The model under review builds one solid part; all positions refer to its coordinate system, in mm. A direction names the side the tool comes from. Coordinates: 2 decimals unless noted, no trailing zeros. Order: outer loops, then holes, each group sorted by start corner. A loop starts at its lowest first (then second) coordinate and runs counter-clockwise, first axis right, second up. Notation, with made-up numbers: M 49,-3.5 L 100,-3.5 A19 ccw 100,14.5 Z; hole C -36.5,73.5 d8. An arc over 180 degrees is marked long. Answer in a Markdown table with one row per item.
from build123d import *

# Parameters (mm, degrees)
ESBO_O1_W                = 175
ESBO_O1_H                = 95
RESSALTO_EXTRUS_O1_DEPTH = 10
ESBO_O2_W                = 6
ESBO_O2_H                = 30
RESSALTO_EXTRUS_O2_DEPTH = 10
ESBO_O3_W                = 6
ESBO_O3_H                = 30
RESSALTO_EXTRUS_O3_DEPTH = 10
ESBO_O4_W                = 30
ESBO_O4_H                = 6
RESSALTO_EXTRUS_O4_DEPTH = 10
ESBO_O5_W                = 30
ESBO_O5_H                = 6
RESSALTO_EXTRUS_O5_DEPTH = 10
ESBO_O7_R                = 1.5
ESBO_O7_R_2              = 1.6
ESBO_O7_R_3              = 6
ESBO_O7_W                = 28.5
ESBO_O7_H                = 22.5
ESBO_O7_W_2              = 15
ESBO_O7_H_2              = 15
ESBO_O7_W_3              = 12
ESBO_O7_H_3              = 12
CORTE_EXTRUS_O2_DEPTH    = 10


with BuildPart() as part:
    # Esboço1 → Ressalto-extrusão1 (new body)
    with BuildSketch(Plane.XY):
        Rectangle(ESBO_O1_W, ESBO_O1_H)
    extrude(amount=RESSALTO_EXTRUS_O1_DEPTH)

    # Esboço2 → Ressalto-extrusão2 (add)
    with BuildSketch(Plane.ZY.offset(87.5)):
        with Locations((5, 0)):
            Rectangle(ESBO_O2_W, ESBO_O2_H)
    extrude(amount=RESSALTO_EXTRUS_O2_DEPTH)

    # Esboço3 → Ressalto-extrusão3 (add)
    with BuildSketch(Plane(origin=(87.5, 0, 0), x_dir=(0, 0, -1), z_dir=(1, 0, 0))):
        with Locations((-5, 0)):
            Rectangle(ESBO_O3_W, ESBO_O3_H)
    extrude(amount=RESSALTO_EXTRUS_O3_DEPTH)

    # Esboço4 → Ressalto-extrusão4 (add)
    with BuildSketch(Plane.XZ.offset(47.5)):
        with Locations((37.5, 5)):
            Rectangle(ESBO_O4_W, ESBO_O4_H)
        with Locations((-37.5, 5)):
            Rectangle(ESBO_O4_W, ESBO_O4_H)
    extrude(amount=RESSALTO_EXTRUS_O4_DEPTH)

    # Esboço5 → Ressalto-extrusão5 (add)
    with BuildSketch(Plane(origin=(0, 47.5, 0), x_dir=(1, 0, 0), z_dir=(0, 1, 0))):
        with Locations((0, -5)):
            Rectangle(ESBO_O5_W, ESBO_O5_H)
    extrude(amount=RESSALTO_EXTRUS_O5_DEPTH)

    # Esboço7 → Corte-extrusão2 (cut)
    with BuildSketch(Plane.XY.offset(10)):
        with Locations((73.5, -34.5)):
            Circle(ESBO_O7_R)
        with Locations((-15.5, -30.5)):
            Circle(ESBO_O7_R)
        with Locations((78.25, 7.25)):
            Circle(ESBO_O7_R_2)
        with Locations((38.25, 7.25)):
            Circle(ESBO_O7_R_2)
        with Locations((-32.5, -17.5)):
            Circle(ESBO_O7_R_3)
        Polygon((72.5, -2.5), (44, -2.5), (44, 11), (49, 17), (67.5, 17), (72.5, 11), align=None)
        with Locations((4.75, 7.25)):
            Rectangle(ESBO_O7_W, ESBO_O7_H)
        with Locations((-71.5, -38)):
            Rectangle(ESBO_O7_W_2, ESBO_O7_H_2)
        with Locations((-41.5, -38)):
            Rectangle(ESBO_O7_W_3, ESBO_O7_H_3)
    extrude(amount=-CORTE_EXTRUS_O2_DEPTH, mode=Mode.SUBTRACT)


solid = part.part
(1) Take a section at D-D (z = 3.75). State how many separate pieces and enclosed holes the cut face has, then the cut area to 3 significant figures.
Report:
| item | result |
|---|---|
| separate pieces | 1 |
| enclosed holes | 9 |
| area | 16,400 mm^2 |
(2) Machinability: for faces 3 (the flat face through (-22.5, -52, 5)), 4 (the flat face through (92, 0, 2)), 5 (the flat face through (-92, -15, 5)), 6 (the flat face through (-72, -45.5, 5)), which of the approach directions +Z, -Z, +X, -X, +Y, -Y give a long, thin tool a straight path to every point of the face, cutting with its end or side? Answer none if there is none.
Report:
| item | result |
|---|---|
| face 3 | +Z, -Z, -Y |
| face 4 | -Z, +X, +Y, -Y |
| face 5 | +Z, -Z, -X, -Y |
| face 6 | +Z, -Z |
(3) Take a section at B-B (y = -17.5). Write out the cut boundary in (x, z).
Report:
| item | result |
|---|---|
| outline | M -87.5,0 L -38.5,0 L -38.5,10 L -87.5,10 Z; M -26.5,0 L 87.5,0 L 87.5,10 L -26.5,10 Z |
(4) To check wall thickness, follow line 1 (X direction, y = 5, z = 6.25); line 2 (X direction, y = 5, z = 9.75); line 3 (X direction, y = 7.5, z = 5.5). State the ranges of each line that lie inside material, in increasing order. Write a range as [from, to].
Report:
| item | result |
|---|---|
| line 1 | [-97.5, -9.5], [19, 44], [72.5, 97.5] |
| line 2 | [-87.5, -9.5], [19, 44], [72.5, 87.5] |
| line 3 | [-97.5, -9.5], [19, 36.67], [39.83, 44], [72.5, 76.67], [79.83, 97.5] |
(5) Take a section at A-A (x = -32.5). Write out the cut boundary in (y, z), then the cut area to 3 significant figures.
Report:
| item | result |
|---|---|
| outline | M -57.5,2 L -47.5,2 L -47.5,0 L -23.5,0 L -23.5,10 L -47.5,10 L -47.5,8 L -57.5,8 Z; M -11.5,0 L 47.5,0 L 47.5,10 L -11.5,10 Z |
| area | 890 mm^2 |
(6) The part is to be moulded in two halves that separate along X. For faces 1 (the flat face through (-42, -32, 5)), 2 (the flat face through (37, -57.5, 5)), say which applies: +X half, -X half, draft (parallel to the pull), parting line (faces both ways), or undercut.
Report:
| item | result |
|---|---|
| face 1 | undercut |
| face 2 | draft |
(7) Take a section at C-C (y = -41). Write out the cut boundary in (x, z), then the cut area to 3 significant figures.
Report:
| item | result |
|---|---|
| outline | M -87.5,0 L -79,0 L -79,10 L -87.5,10 Z; M -64,0 L -47.5,0 L -47.5,10 L -64,10 Z; M -35.5,0 L 87.5,0 L 87.5,10 L -35.5,10 Z |
| area | 1,480 mm^2 |
(8) Insertion check: P1, Ø5, axis at x = -69, z = 4, coming from the +Y side; P2, Ø5, axis at y = 53.5, z = 5.5, coming from the -X side; P3, Ø10, axis at x = 51, y = -14.5, coming from the -Z side; P4, Ø2.5, axis at x = 38.25, y = 7.25, coming from the +Z side. Each pin has a flat end and moves straight along its axis. Give the tip position at first contact, or say it passes through.
Report:
| item | result |
|---|---|
| P1 | y = 47.5 |
| P2 | x = -15 |
| P3 | z = 0 |
| P4 | through |
